```python
from build123d import *

# Parameters (mm, degrees)
SKETCH1_R                       = 10.5
BOSS_EXTRUDE1_DEPTH             = 1.5
CUT_EXTRUDE1_DEPTH              = 15.924811557
CUT_EXTRUDE1_DEPTH_BACK         = 15.924811557
SKETCH2_R                       = 0.8
M2_CLEARANCE_HOLE1_D            = 2.2
M2_CLEARANCE_HOLE1_DEPTH        = 5
M2_CLEARANCE_HOLE1_TIP          = 0.660946681
BOSS_EXTRUDE2_START             = 3
SKETCH7_R                       = 10.5
SKETCH7_R_2                     = 7.2
BOSS_EXTRUDE2_DEPTH             = 3
FILLET1_R                       = 1
CHAMFER1_SIZE                   = 1
CHAMFER2_SIZE                   = 1
M2X0_4_TAPPED_HOLE1_D           = 1.6
M2X0_4_TAPPED_HOLE1_DEPTH       = 5.2
M2X0_4_TAPPED_HOLE1_CSINK_D     = 2.05
M2X0_4_TAPPED_HOLE1_CSINK_ANGLE = 90
M2X0_4_TAPPED_HOLE1_TIP         = 0.480688495


with BuildPart() as part:
    # Sketch1 → Boss-Extrude1 (new body)
    with BuildSketch(Plane(origin=(0, 0, 0), x_dir=(1, 0, 0), z_dir=(0, 1, 0))):
        with Locations(Location((0, 0, 0), (0, 0, 270))):
            Circle(SKETCH1_R)
    extrude(amount=BOSS_EXTRUDE1_DEPTH)

    # Sketch2 → Cut-Extrude1 (cut, two sides: drawn at the far end of the back side and taken through both)
    with BuildSketch(Plane(origin=(0, 1.5, 0), x_dir=(1, 0, 0), z_dir=(0, 1, 0)).offset(-CUT_EXTRUDE1_DEPTH_BACK)):
        with Locations(Location((0, 0, 0), (0, 0, 270))):
            Circle(SKETCH2_R)
    extrude(amount=CUT_EXTRUDE1_DEPTH + CUT_EXTRUDE1_DEPTH_BACK, mode=Mode.SUBTRACT)

    # M2 Clearance Hole1
    with Locations(Plane(origin=(0, 1.5, 0), x_dir=(1, 0, 0), z_dir=(0, 1, 0))):
        with Locations((-1.767766953, 1.767766953), (1.767766953, 1.767766953), (1.767766953, -1.767766953), (-1.767766953, -1.767766953)):
            Hole(M2_CLEARANCE_HOLE1_D / 2, depth=M2_CLEARANCE_HOLE1_DEPTH)
            with Locations((0, 0, -(M2_CLEARANCE_HOLE1_DEPTH + M2_CLEARANCE_HOLE1_TIP / 2))):  # 118° drill point
                Cone(0, M2_CLEARANCE_HOLE1_D / 2, M2_CLEARANCE_HOLE1_TIP, mode=Mode.SUBTRACT)

    # Sketch6 → Revolve1 (revolve)
    with BuildSketch(Plane.XY, mode=Mode.PRIVATE) as revolve1_sk:
        Polygon((-10.5, 0), (-10.5, -1.25), (-7.2, -1.25), (-5, 0), align=None)
    revolve(revolve1_sk.sketch.rotate(Axis((0, 0, 0), (0, -1, 0)), 270), axis=Axis((0, 0, 0), (0, -1, 0)))

    # Sketch7 → Boss-Extrude2 (add)
    with BuildSketch(Plane.XZ.offset(1.25).offset(BOSS_EXTRUDE2_START)):
        with Locations(Location((0, 0, 0), (0, 0, 270))):
            Circle(SKETCH7_R)
        with Locations(Location((0, 0, 0), (0, 0, 90))):
            Circle(SKETCH7_R_2, mode=Mode.SUBTRACT)
    extrude(amount=-BOSS_EXTRUDE2_DEPTH)

    # Fillet1
    fillet1_edges = [part.edges().sort_by_distance(p)[0] for p in [
        (0, -1.25, -7.2),
        (0, 0, -5),
    ]]
    fillet(fillet1_edges, radius=FILLET1_R)

    # Chamfer1
    # the kernel refuses this chamfer: 1 mm, written as the material it takes off along each edge
    with BuildSketch(Plane(origin=(0, 1.5, 0), x_dir=(0, 0, 1), z_dir=(-1, 0, 0))) as chamfer1_piece_1:
        Polygon((10.5, -CHAMFER1_SIZE), (10.5 - CHAMFER1_SIZE, 0), (10.5, 0), align=None)
    revolve(axis=Axis((0, 1.5, 0), (0, 1, 0)), mode=Mode.SUBTRACT)

    # Chamfer2
    chamfer2_edges = [part.edges().sort_by_distance(p)[0] for p in [
        (0, -4.25, 10.5),
    ]]
    chamfer(chamfer2_edges, length=CHAMFER2_SIZE)

    # M2x0.4 Tapped Hole1
    with Locations(Plane(origin=(0, 1.5, 0), x_dir=(1, 0, 0), z_dir=(0, 1, 0))):
        with Locations((-3.889087297, 3.889087297), (3.889087297, -3.889087297), (-1.767766953, 1.767766953)):
            CounterSinkHole(M2X0_4_TAPPED_HOLE1_D / 2, M2X0_4_TAPPED_HOLE1_CSINK_D / 2, depth=M2X0_4_TAPPED_HOLE1_DEPTH, counter_sink_angle=M2X0_4_TAPPED_HOLE1_CSINK_ANGLE)
            with Locations((0, 0, -(M2X0_4_TAPPED_HOLE1_DEPTH + M2X0_4_TAPPED_HOLE1_TIP / 2))):  # 118° drill point
                Cone(0, M2X0_4_TAPPED_HOLE1_D / 2, M2X0_4_TAPPED_HOLE1_TIP, mode=Mode.SUBTRACT)


solid = part.part
```
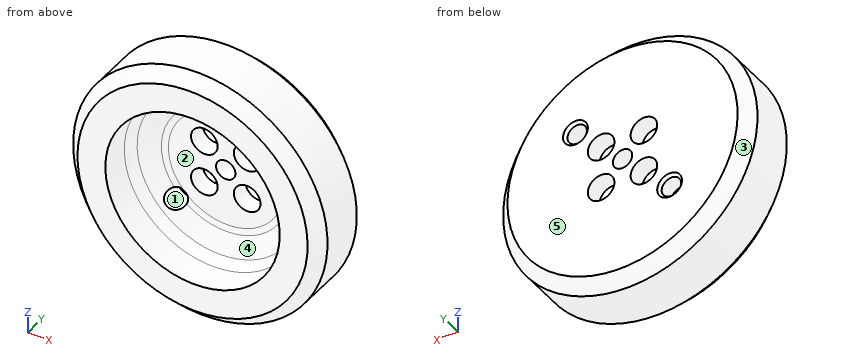
Work out the finished part from the listing and answer in its coordinate system (mm). Face numbers are marked on the shaded views. A direction names the side the tool comes from. Give positions to 0.01 mm unless a question says otherwise; leave off trailing zeros. Loops run counter-clockwise (first coordinate to the right, second up) from the corner with the lowest first, then second, coordinate; pieces in that order, holes last. Notation, with made-up numbers: M -13,69.5 L 7,69.5 A36 cw 7,104.5 Z; hole C 87,57.25 d10. An arc over 180 degrees is marked long. One line per item, written item: value. Start each with the question number.
1. Determine the mould class of the marked faces 3, 4 and 5 for opening direction X: released by +X, released by -X, zero draft, split by the parting line, or undercut.
2. Which of the six approach directions +Z, -Z, +X, -X, +Y, -Y give full straight-line access (tool end or side, diameter ignored) to the marked faces 1 and 2?
3. Find section A-A (y = -2.5). Give the vertices of the cut face in (x, z).
4. Each of these flat-tipped pins is pushed along its axis until it touches: P1, Ø4.5, axis at x = -2, z = 0.5, coming from the -Y side; P2, Ø1.5, axis at y = 0, z = 6.5, coming from the +X side; P3, Ø3, axis at y = 0, z = -4.5, coming from the -X side. Where does it stop, or does it pass through?
5. Find the intervals of material crossed by probe 1 along X at (y, z) = (-1.8, -0.25); probe 2 along X at (y, z) = (0.45, 0); probe 3 along Y at (x, z) = (-3.5, 0), in increasing order.
Reported:
1. face 3: split by the parting line
1. face 4: undercut
1. face 5: zero draft
2. face 1: +Y, -Y
2. face 2: -Y
3. outline: C 0,0 d21; hole C 0,0 d14.4
4. P1: stops at y = 0
4. P2: stops at x = 8.79
4. P3: stops at x = -10.06
5. probe 1: x = -10.5 to -7.2, 7.2 to 10.5
5. probe 2: x = -10.5 to -0.8, 0.8 to 10.5
5. probe 3: y = 0 to 1.5
